Part model, mm, in its own coordinate system. A direction names the side the tool comes from. Give positions to 0.01 mm unless a question says otherwise; leave off trailing zeros. Return JSON: item names as keys, results as strings.
Autodesk Inventor part; units mm, degrees
ref_plane "Płaszczyzna konstrukcyjna1" through (64.95, 71.5, 0) normal (1, 0, 0) x (0, 1, 0)
ref_plane "Płaszczyzna konstrukcyjna2" through (0, 0, 29) normal (0, 0, 1) x (1, 0, 0)
ref_plane "XZ Plane" through (0, 0, 0) normal (0, 1, 0) x (-1, 0, 0)
sketch "Szkic2" plane through (0, 0, 0) normal (0, 0, 1) x (1, 0, 0)
  line L0 (4.75, 102.75) -> (9.25, 102.75)
  line L1 (9.25, 102.75) -> (9.25, 107.25)
  line L2 (9.25, 107.25) -> (4.75, 107.25)
  line L3 (4.75, 107.25) -> (4.75, 102.75)
  line L4 (4.75, 102.75) -> (9.25, 107.25) construction
  line L5 (9.25, 102.75) -> (4.75, 107.25) construction
  point P0 (0, 0)
  point P1 (64.95, 71.5)
  point P2 (7, 105)
  dimension "d1" = 4.5
  dimension "d2" = 4.5
ref_plane "Płaszczyzna konstrukcyjna1" through (64.95, 71.5, 0) normal (1, 0, 0) x (0, 1, 0)
ref_plane "Płaszczyzna konstrukcyjna2" through (0, 0, 29) normal (0, 0, 1) x (1, 0, 0)
sketch "Szkic3" plane through (0, 0, 29) normal (0, 0, 1) x (1, 0, 0)
  circle A0 centre (40.75, 71) radius 1.75
  point P0 (0, 0)
extrude "Wyciągnięcie proste1" add sketch "Szkic2" against normal blind 6
sketch "Szkic4" plane through (0, 0, 0) normal (0, 0, 1) x (1, 0, 0)
  line L0 (4.75, 102.75) -> (9.25, 102.75)
  line L1 (9.25, 102.75) -> (9.25, 107.25)
  line L2 (9.25, 107.25) -> (4.75, 107.25)
  line L3 (4.75, 107.25) -> (4.75, 102.75)
  point P0 (0, 0)
sketch "Szkic5" plane through (0, 0, 29) normal (0, 0, 1) x (1, 0, 0)
  line L0 (64.95, 149.0685) -> (64.95, -24.8448) construction
  line L1 (64.95, 88) -> (64.95, 96) construction
  line L2 (64.95, 96) -> (47.95, 96) construction
  circle A0 centre (47.95, 96) radius 2
  line L3 (64.95, 96) -> (64.95, 84) construction
  line L4 (64.95, 84) -> (57.7389, 84) construction
  arc A1 (64.95, 110) -> (57.7389, 84) centre (64.95, 96) ccw
  line L5 (57.7389, 84) -> (57.7389, 79)
  line L6 (57.7389, 79) -> (64.95, 79)
  circle A2 centre (40.75, 71) radius 1.75
  line L7 (64.95, 96) -> (81.95, 96) construction
  circle A3 centre (81.95, 96) radius 2
  line L8 (64.95, 84) -> (72.1611, 84) construction
  arc A4 (72.1611, 84) -> (64.95, 110) centre (64.95, 96) ccw
  line L9 (72.1611, 84) -> (72.1611, 79)
  line L10 (72.1611, 79) -> (64.95, 79)
  circle A5 centre (89.15, 71) radius 1.75
  arc A6 (36.75, 71) -> (44.75, 71) centre (40.75, 71) ccw
  arc A7 (85.15, 71) -> (93.15, 71) centre (89.15, 71) ccw
  arc A8 (85.15, 71) -> (44.75, 71) centre (64.95, 34.5448) ccw
  spline S0 degree 3 poles (4.75, 99.25) (3.3447, 87.1152) (30.6878, 94.0489) (36.75, 71) knots 0 0 0 0 1 1 1 1
  spline S1 degree 3 poles (125.15, 99.25) (126.5553, 87.1152) (99.2122, 94.0489) (93.15, 71) knots 0 0 0 0 1 1 1 1
  spline S2 degree 4 poles (4.75, 107.25) (7.6598, 112.7952) (35.9373, 119.5714) (52.5371, 120.1837) (64.95, 120.886) knots 0 0 0 0 0 1 1 1 1 1
  spline S3 degree 4 poles (125.15, 107.25) (122.2402, 112.7952) (93.9627, 119.5714) (77.3629, 120.1837) (64.95, 120.886) knots 0 0 0 0 0 1 1 1 1 1
  line L11 (125.15, 107.25) -> (125.15, 99.25)
  line L12 (4.75, 107.25) -> (4.75, 99.25)
  point P0 (0, 0)
  point P1 (50.95, 96)
  point P2 (78.95, 96)
  point P3 (7.7703, 93.2829)
  point P4 (21.1067, 88)
  point P5 (122.1297, 93.2829)
  point P6 (108.7933, 88)
  point P7 (10.3549, 111.0646)
  point P8 (29.8942, 116.7506)
  point P9 (51.4593, 119.9555)
  point P10 (119.5451, 111.0646)
  point P11 (100.0058, 116.7506)
  point P12 (78.4407, 119.9555)
  dimension "d7" = 17
  dimension "d8" = 4
  dimension "d9" = 12
  dimension "d10" = 5
  dimension "d13" = 4
  dimension "d14" = 8
extrude "Wyciągnięcie proste2" add sketch "Szkic5" along normal blind 8
sketch "Szkic6" plane through (0, 0, 29) normal (0, 0, -1) x (-1, 0, 0)
  line L0 (-9.25, 107.25) -> (-4.75, 107.25)
  line L1 (-4.75, 107.25) -> (-4.75, 99.25)
  line L2 (-4.75, 107.25) -> (-14.75, 107.25)
  line L3 (-14.75, 107.25) -> (-14.75, 99.25)
  line L4 (-14.75, 99.25) -> (-4.75, 99.25)
  line L5 (-4.75, 99.25) -> (-4.75, 107.25)
  line L6 (-64.95, -24.1772) -> (-64.95, 145.0632) construction
  point P0 (0, 0)
  point P1 (-125.15, 107.25)
  dimension "d19" = 10
  dimension "d20" = 8
sketch "Szkic7" plane through (0, 0, 0) normal (0, 0, 1) x (1, 0, 0)
  line L0 (4.75, 102.75) -> (9.25, 102.75)
  line L1 (9.25, 102.75) -> (9.25, 107.25)
  line L2 (9.25, 107.25) -> (4.75, 107.25)
  line L3 (4.75, 107.25) -> (4.75, 102.75)
  line L4 (4.75, 102.75) -> (9.25, 102.75)
  line L5 (4.75, 102.75) -> (9.25, 102.75)
  line L6 (9.25, 102.75) -> (9.25, 107.25)
  line L7 (9.25, 107.25) -> (4.75, 107.25)
  line L8 (4.75, 107.25) -> (4.75, 102.75)
  point P0 (0, 0)
  dimension "d21" = 4.5
  dimension "d22" = 4.5
loft "Wyciągnięcie złożone1" add profiles "Szkic6" section 1 edges at (7, 102.75, 0) (9.25, 105, 0) (7, 107.25, 0) (4.75, 105, 0)
mirror "Odbij1" about plane through (64.95, 71.5, 0) normal (1, 0, 0) of "Wyciągnięcie złożone1", "Wyciągnięcie proste1"
properties part number "turret_base"
Q1. Probe line 1 along X through (y, z) = (71, 33); line 2 along Z through (x, y) = (77.5, 108); line 3 along Y through (x, z) = (81.95, 33.75). List the from-to ranges inside material, lowest first.
Established:
{"line 1": "x = 36.75 to 39, 42.5 to 44.75, 85.15 to 87.4, 90.9 to 93.15", "line 2": "z = 29 to 37", "line 3": "y = 72.6 to 94, 98 to 119.6"}
Q2. 3-axis set-ups, long thin cutter, end or side, ignore diameter. For faces 4 (the flat face through (120.65, 105, -3)), 5 (the flat face through (72.161, 82, 33)), 6 (the flat face through (7, 102.75, -3)), 7 (the flat face through (8, 107.25, 16)): which of +Z, -Z, +X, -X, +Y, -Y reach the whole face in a straight line?
Established:
{"face 4": "-Z, +Y, -Y", "face 5": "+Z, -Z", "face 6": "-Z, +X, -X, -Y", "face 7": "-Z, +X, -X, +Y"}
Q3. Pin check, flat tips, straight feed: pin 1 (3.5 mm diameter, centred on y = 106, z = -2, fed in from +X); pin 2 (5 mm diameter, centred on y = 104.5, z = -4.5, fed in from -X); pin 3 (8 mm diameter, centred on x = 8, z = 13.5, fed in from +Y). Stop position of each tip, or through.
Established:
{"pin 1": "stops at x = 125.15", "pin 2": "stops at x = 4.75", "pin 3": "stops at y = 107.25"}
Q4. Two-plate mould, pull along Y, no slides. Class faces 1 (the flat face through (123, 102.75, -3)), 2 (the flat face through (9.25, 105, -3)), 3 (the cylindrical face through (87.76, 72.06, 32.94)): +Y half, -Y half, draft (parallel to the pull), parting line (faces both ways), or undercut.
Established:
{"face 1": "-Y half", "face 2": "draft", "face 3": "undercut"}
